The model under review builds one solid part; all positions refer to its coordinate system, in mm. A direction names the side the tool comes from. Round coordinates to 2 decimals unless told otherwise and drop trailing zeros. Write each loop counter-clockwise with the first axis right and the second up, starting at its lowest first coordinate (ties: lowest second). Pieces come first, ordered by that corner, then holes. Notation, with made-up numbers: (-14, 4.25) - (9, 4.25) arc R21 ccw to (9, 11.25) - close; hole circle Ø9 at (-4, 14.25). An arc over 180 degrees is marked (long way). Write each question's results on one line, items separated by ' | '.
```python
from build123d import *

# Parameters (mm, degrees)
F0_R     = 2.5
F1_DEPTH = 3
F3_DEPTH = 4
F4_R     = 1
F5_DEPTH = 4


with BuildPart() as f1:
    # F0 (on Front) → F1 (new body)
    with BuildSketch(Plane.XZ):
        Circle(F0_R)
    extrude(amount=F1_DEPTH)

    # F2 (on face) → F3 (join)
    with BuildSketch(Plane.XZ.offset(3)):
        with BuildLine():
            Line((1.920937, 1.6), (-1.920937, 1.6))
            ThreePointArc((-1.920937, 1.6), (-2.5, 0), (-1.920937, -1.6))
            Line((-1.920937, -1.6), (1.920937, -1.6))
            ThreePointArc((1.920937, -1.6), (2.350781, -0.850781), (2.5, 0))
            ThreePointArc((2.5, 0), (2.350781, 0.850781), (1.920937, 1.6))
        make_face()
    extrude(amount=F3_DEPTH)

    # F4 (on face) → F5 (cut)
    with BuildSketch(Plane.XZ.offset(7)):
        Circle(F4_R)
    extrude(amount=-F5_DEPTH, mode=Mode.SUBTRACT)


solid = f1.part
```
Q1. We need section A-A (x = 0). State the section outline as (y, z) points, plus the area to 3 significant figures.
Evaluation:
outline: (-7, -1.6) - (-3, -1.6) - (-3, -2.5) - (0, -2.5) - (0, 2.5) - (-3, 2.5) - (-3, 1.6) - (-7, 1.6) - (-7, 1) - (-3, 1) - (-3, -1) - (-7, -1) - close | area: 19.8 mm^2
Q2. The part is to be moulded in two halves that separate along Z. For faces 6 (the flat face through (0, -5, -1.6)), 7 (the flat face through (0, -3, 0)), 8 (the flat face through (0, -3, 2)), say which applies: released by +Z, released by -Z, zero draft, split by the parting line, or undercut.
Evaluation:
face 6: released by -Z | face 7: undercut | face 8: zero draft
Q3. We need section D-D (y = -2). State the section outline as (x, z) points.
Evaluation:
outline: circle Ø5 at (0, 0)
Q4. Tool access review of faces 1 (the flat face through (0, 0, 0)), 2 (the cylindrical face through (0, -5, -1)), 3 (the flat face through (1.1, -7, 0.4)), 4 (the flat face through (0, -3, -2)), 5 (the flat face through (0, -5, 1.6)): name each direction out of +Z, -Z, +X, -X, +Y, -Y from which nothing blocks a thin tool from reaching the whole face with its end or side.
Evaluation:
face 1: +Z, -Z, +X, -X, +Y | face 2: -Y | face 3: +Z, -Z, +X, -X, -Y | face 4: -Z, +X, -X, -Y | face 5: +Z, +X, -X, -Y
Q5. For probe 1 along Z at (x, y) = (0, -4.85); probe 2 along Z at (x, y) = (-1.65, -4.5); probe 3 along Y at (x, z) = (-1, -1.9), list the stretches that pass through material, from the lowest coordinate up.
Evaluation:
probe 1: z = -1.6 to -1, 1 to 1.6 | probe 2: z = -1.6 to 1.6 | probe 3: y = -3 to 0
Q6. We need section C-C (z = 0.6). State the section outline as (x, y) points.
Evaluation:
outline: (-2.43, -7) - (-0.8, -7) - (-0.8, -3) - (0.8, -3) - (0.8, -7) - (2.43, -7) - (2.43, 0) - (-2.43, 0) - close
Q7. Insertion check: P1, Ø1, axis at y = -5.5, z = -1.5, coming from the -X side; P2, Ø1.5, axis at y = -5.5, z = 1, coming from the +X side; P3, Ø1.9, axis at x = -0.5, y = -5, coming from the -Z side. Each pin has a flat end and moves straight along its axis. Give the tip position at first contact, or say it passes through.
Evaluation:
P1: stops at x = -2.29 | P2: stops at x = 2.49 | P3: stops at z = -1.6
Q8. We need section B-B (y = -6.5). State the section outline as (x, z) points.
Evaluation:
outline: (-1.92, -1.6) - (1.92, -1.6) arc R2.5 ccw to (1.92, 1.6) - (-1.92, 1.6) arc R2.5 ccw to start; hole circle Ø2 at (0, 0)
